from build123d import *

# Parameters (mm, degrees)
F0_W     = 114.3
F0_H     = 266.7
F2_DEPTH = 25.4
F1_R     = 6.35
F1_R_2   = 19.05
F3_DEPTH = 25.4
F5_R     = 6.35
F6_DEPTH = 25.4


with BuildPart() as f2:
    # F0 (on Front) → F2 (new body)
    with BuildSketch(Plane.XZ):
        with Locations((-57.15, 133.35)):
            Rectangle(F0_W, F0_H)
    extrude(amount=F2_DEPTH)

    # F1 (on face) → F3 (cut)
    with BuildSketch(Plane.XZ):
        with BuildLine():
            ThreePointArc((-66.675, 50.8), (-73.025, 57.15), (-79.375, 50.8))
            ThreePointArc((-79.375, 50.8), (-73.025, 44.45), (-66.675, 50.8))
        make_face()
        with BuildLine():
            ThreePointArc((-88.9, 44.45), (-107.95, 25.4), (-88.9, 6.35))
            Line((-88.9, 6.35), (-88.9, 25.4))
            Line((-88.9, 25.4), (-88.9, 44.45))
        make_face()
        with BuildLine():
            Line((-88.9, 25.4), (-88.9, 6.35))
            ThreePointArc((-88.9, 6.35), (-75.429616, 11.929616), (-69.85, 25.4))
            ThreePointArc((-69.85, 25.4), (-75.429616, 38.870384), (-88.9, 44.45))
            Line((-88.9, 44.45), (-88.9, 25.4))
        make_face()
        with BuildLine():
            ThreePointArc((-38.1, 76.2), (-70.620384, 89.670384), (-57.15, 57.15))
            ThreePointArc((-57.15, 57.15), (-43.679616, 62.729616), (-38.1, 76.2))
        make_face()
        with Locations((-41.275, 50.8)):
            Circle(F1_R)
        with BuildLine():
            ThreePointArc((-25.4, 44.45), (-44.45, 25.4), (-25.4, 6.35))
            Line((-25.4, 6.35), (-25.4, 25.4))
            Line((-25.4, 25.4), (-25.4, 44.45))
        make_face()
        with BuildLine():
            Line((-25.4, 25.4), (-25.4, 6.35))
            ThreePointArc((-25.4, 6.35), (-11.929616, 11.929616), (-6.35, 25.4))
            ThreePointArc((-6.35, 25.4), (-11.929616, 38.870384), (-25.4, 44.45))
            Line((-25.4, 44.45), (-25.4, 25.4))
        make_face()
        with Locations((-73.025, 101.6)):
            Circle(F1_R)
        with Locations((-41.275, 101.6)):
            Circle(F1_R)
        with Locations((-73.025, 152.4)):
            Circle(F1_R)
        with Locations((-41.275, 152.4)):
            Circle(F1_R)
        with Locations((-88.9, 127)):
            Circle(F1_R_2)
        with Locations((-25.4, 127)):
            Circle(F1_R_2)
        with Locations((-73.025, 203.2)):
            Circle(F1_R)
        with Locations((-41.275, 203.2)):
            Circle(F1_R)
        with Locations((-57.15, 177.8)):
            Circle(F1_R_2)
        with Locations((-88.9, 228.6)):
            Circle(F1_R_2)
        with Locations((-25.4, 228.6)):
            Circle(F1_R_2)
    extrude(amount=F3_DEPTH, mode=Mode.SUBTRACT)

    # F5 (on face) → F6 (cut)
    with BuildSketch(Plane.XZ.offset(25.4)):
        with BuildLine():
            ThreePointArc((-79.375, 76.2), (-90.215128, 80.690128), (-85.725, 69.85))
            ThreePointArc((-85.725, 69.85), (-81.234872, 71.709872), (-79.375, 76.2))
        make_face()
        with BuildLine():
            ThreePointArc((-50.8, 25.4), (-61.640128, 29.890128), (-57.15, 19.05))
            ThreePointArc((-57.15, 19.05), (-52.659872, 20.909872), (-50.8, 25.4))
        make_face()
        with BuildLine():
            ThreePointArc((-22.225, 76.2), (-33.065128, 80.690128), (-28.575, 69.85))
            ThreePointArc((-28.575, 69.85), (-24.084872, 71.709872), (-22.225, 76.2))
        make_face()
        with Locations((-85.725, 177.8)):
            Circle(F5_R)
        with Locations((-28.575, 177.8)):
            Circle(F5_R)
        with Locations((-57.15, 127)):
            Circle(F5_R)
        with Locations((-57.15, 228.6)):
            Circle(F5_R)
    extrude(amount=-F6_DEPTH, mode=Mode.SUBTRACT)


solid = f2.part
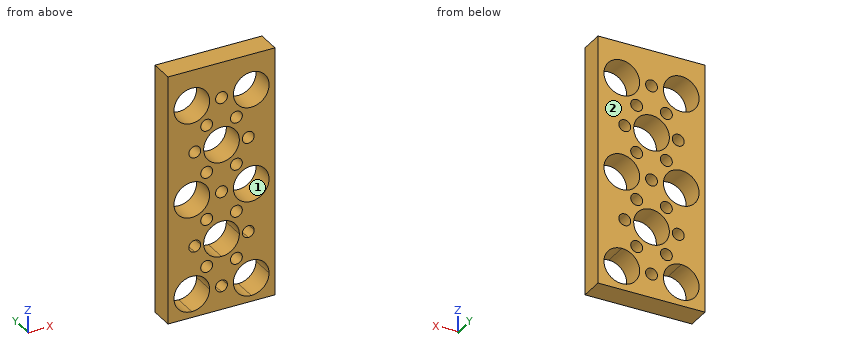
Work out the finished part from the listing and answer in its coordinate system (mm). Face numbers are marked on the shaded views. Give positions to 0.01 mm unless a question says otherwise; leave off trailing zeros. Write each loop counter-clockwise with the first axis right and the second up, starting at its lowest first coordinate (ties: lowest second). Pieces come first, ordered by that corner, then holes. Notation, with made-up numbers: (58, 38.25) - (87, 38.25) arc R14 cw to (87, 54.25) - close; hole circle Ø7 at (10.25, -3). An arc over 180 degrees is marked (long way). One line per item, written item: value. Start each with the question number.
1. Find section C-C (z = 186.5). Write down the section's boundary in (x, y), then the cut area to 3 significant figures.
2. Find section D-D (y = -13.75). State how many separate pieces and enclosed holes the cut face has, then the cut area to 3 significant figures.
3. Consider probe 1 along X at (y, z) = (-19.75, 50.5); probe 2 along Z at (x, y) = (-25, -13); probe 3 along Z at (x, y) = (-25.5, -7.5). Determine where each line is inside the solid, lowest interval first.
4. For a pull along Z with two mould halves and no side action, classify the marked faces 1 and 2 as +Z half, -Z half, draft (parallel to the pull), parting line (faces both ways), or undercut.
5. Given pin 1 (23 mm diameter, centred on x = -88.9, z = 228.6, fed in from -Y), flat-ended and moving along its own axis, determine where the tip first touches the part or whether it passes through.
6. Find section A-A (z = 228.6). Write down the section's boundary in (x, y), then the cut area to 3 significant figures.
7. Find section B-B (x = -17.5). Write down the section's boundary in (y, z).
Geometry results:
1. outline: (-114.3, -25.4) - (-74.1, -25.4) - (-74.1, 0) - (-114.3, 0) - close; (-40.2, -25.4) - (0, -25.4) - (0, 0) - (-40.2, 0) - close
1. area: 2,040 mm2
2. separate pieces: 1
2. enclosed holes: 23
2. area: 19,500 mm2
3. probe 1: -114.3 to -79.37, -66.68 to -47.62, -34.93 to 0
3. probe 2: 0 to 6.35, 44.45 to 70.95, 81.45 to 107.95, 146.05 to 172.55, 183.05 to 209.55, 247.65 to 266.7
3. probe 3: 0 to 6.35, 44.45 to 70.64, 81.76 to 107.95, 146.05 to 172.24, 183.36 to 209.55, 247.65 to 266.7
4. face 1: undercut
4. face 2: draft
5. pin 1: through
6. outline: (-114.3, -25.4) - (-107.95, -25.4) - (-107.95, 0) - (-114.3, 0) - close; (-69.85, -25.4) - (-63.5, -25.4) - (-63.5, 0) - (-69.85, 0) - close; (-50.8, -25.4) - (-44.45, -25.4) - (-44.45, 0) - (-50.8, 0) - close; (-6.35, -25.4) - (0, -25.4) - (0, 0) - (-6.35, 0) - close
6. area: 645 mm2
7. outline: (-25.4, 0) - (0, 0) - (0, 8.07) - (-25.4, 8.07) - close; (-25.4, 42.73) - (0, 42.73) - (0, 109.67) - (-25.4, 109.67) - close; (-25.4, 144.33) - (0, 144.33) - (0, 211.27) - (-25.4, 211.27) - close; (-25.4, 245.93) - (0, 245.93) - (0, 266.7) - (-25.4, 266.7) - close
